Verification items for the finished model (mm, model axes). A direction names the side the tool comes from. Round coordinates to 2 decimals unless told otherwise and drop trailing zeros. Write each loop counter-clockwise with the first axis right and the second up, starting at its lowest first coordinate (ties: lowest second). Pieces come first, ordered by that corner, then holes. Notation, with made-up numbers: (-4.5, 86.5) - (21.5, 86.5) arc R13 ccw to (21.5, 102.5) - close; hole circle Ø1 at (16, -2). An arc over 180 degrees is marked (long way). Answer as a JSON object with one key per item and string values. Group by question number.
1) Thickness scan on line 1 (Y direction, x = 1.5, z = 7.25); line 2 (Z direction, x = 10.75, y = 1.5); line 3 (X direction, y = -21, z = -0.5). Record the ranges inside material, lowest first.
2) Section check B-B (x = 2.5). Enter the section's corners in (y, z).
3) Section check D-D (z = -8.5). Enter the section's corners in (x, y).
4) Set-up check for faces 1 (the cylindrical face through (-6, -54, 0)), 2 (the flat face through (-9.43, 4.93, 6.835)): record each of +Z, -Z, +X, -X, +Y, -Y from which the full face is reachable in a straight line by a thin tool's end or side.
5) Section check C-C (y = -35). Enter the section's corners in (x, z), then the cut area to 3 significant figures.
6) Go/stop test with flat-tipped pins: pin 1 Ø6 at (x, y) = (9.5, -33.5) entering from -Z; pin 2 Ø2 at (x, y) = (-2.5, -96) entering from -Z; pin 3 Ø5 at (y, z) = (-84.5, 0.5) entering from +X; pin 4 Ø6 at (y, z) = (-93, 7.5) entering from +X. Record where each tip stops, or that it passes through.
7) Section check A-A (z = 4.5). Enter the section's corners in (x, y), then the cut area to 3 significant figures.
```python
from build123d import *

# Parameters (mm, degrees)
BOSS_EXTRUDE1_DEPTH = 10
SKETCH2_R           = 6
BOSS_EXTRUDE2_DEPTH = 110


with BuildPart() as part:
    # Sketch1 → Boss-Extrude1 (new body)
    with BuildSketch(Plane(origin=(0, 0, 0), x_dir=(1, 0, 0), z_dir=(0, 1, 0))):
        Polygon((7.979415777, -10.824700142), (13.3641732, 1.498026699), (5.384757423, 12.322726841), (-7.979415777, 10.824700142), (-13.3641732, -1.498026699), (-5.384757423, -12.322726841), align=None)
    extrude(amount=BOSS_EXTRUDE1_DEPTH)

    # Sketch2 → Boss-Extrude2 (add)
    with BuildSketch(Plane.XZ):
        Circle(SKETCH2_R)
    extrude(amount=BOSS_EXTRUDE2_DEPTH)


solid = part.part
```
Returned:
{
 "1": {"line 1": "0 to 10", "line 2": "-5.04 to 4.48", "line 3": "-5.98 to 5.98"},
 "2": {"outline": "(-110, -5.45) - (0, -5.45) - (0, -12) - (10, -12) - (10, 11.44) - (0, 11.44) - (0, 5.45) - (-110, 5.45) - close"},
 "3": {"outline": "(-9, 0) - (8.2, 0) - (8.2, 10) - (-9, 10) - close"},
 "4": {"face 1": "-Y", "face 2": "+Z, -X, +Y, -Y"},
 "5": {"outline": "circle Ø12 at (0, 0)", "area": "113 mm2"},
 "6": {"pin 1": "through", "pin 2": "z = -5.81", "pin 3": "x = 6", "pin 4": "x = 3.97"},
 "7": {"outline": "(-11.15, 0) - (-3.97, 0) - (-3.97, -110) - (3.97, -110) - (3.97, 0) - (10.74, 0) - (10.74, 10) - (-11.15, 10) - close", "area": "1,090 mm2"}
}
